Build history of the part. All positions in model axes, mm. Round coordinates to 2 decimals unless told otherwise and drop trailing zeros. Order: outer loops, then holes, each group sorted by start corner. A loop starts at its lowest first (then second) coordinate and runs counter-clockwise, first axis right, second up. Notation, with made-up numbers: M -27.75,42.25 L -6.75,42.25 A23 cw -6.75,67.25 Z; hole C 18.5,-8 d8. An arc over 180 degrees is marked long. One line per item, written item: value. Start each with the question number.
Item 1: Band-saw the part on B-B, the plane y = -2.25. Write the cut outline in (x, z), then the cut area to 3 significant figures.
Item 2: Probe L1, parallel to X at y = 2.5, z = 2.75; L2, parallel to X at y = 2.5, z = 0; L3, parallel to Y at x = -7.75, z = -4. List the from-to ranges inside material, lowest first.
Item 3: Pin check, flat tips, straight feed: pin 1 (1.5 mm diameter, centred on x = 5, y = 2, fed in from -Z); pin 2 (1.5 mm diameter, centred on y = 0, z = 6.5, fed in from +X); pin 3 (4 mm diameter, centred on x = 3.5, y = 2.5, fed in from +Z). Stop position of each tip, or through.
Item 4: Band-saw the part on A-A, the plane y = -0.5. Write the cut outline in (x, z), then the cut area to 3 significant figures.
Item 5: Two-plate mould, pull along Z, no slides. Class faces 1 (the flat face through (-4.6, 3.5, 7.5)), 2 (the cylindrical face through (-2.58, 2.51, -8.18)): +Z half, -Z half, draft (parallel to the pull), parting line (faces both ways), or undercut.
```python
from build123d import *

# Parameters (mm, degrees)
CUT_EXTRUDE1_DEPTH      = 16.720209922
CUT_EXTRUDE1_DEPTH_BACK = 16.720209922
SKETCH3_W               = 21.5
SKETCH3_H               = 0.5


with BuildPart() as part:
    # Sketch2 → Revolve1 (revolve)
    with BuildSketch(Plane.XY, mode=Mode.PRIVATE) as revolve1_sk:
        with BuildLine():
            Line((8.578101022, -1.538329541), (8.578101022, -4))
            Line((8.578101022, -4), (9.978101022, -4))
            ThreePointArc((9.978101022, -4), (10.75, 0), (9.978101022, 4))
            Line((9.978101022, 4), (8.578101022, 4))
            Line((8.578101022, 4), (8.578101022, 1.538329541))
            ThreePointArc((8.578101022, 1.538329541), (9.110552684, 0.849646384), (9.3, 0))
            ThreePointArc((9.3, 0), (9.110552684, -0.849646384), (8.578101022, -1.538329541))
        make_face()
    revolve(revolve1_sk.sketch.rotate(Axis((0, 0, 0), (0, 1, 0)), 90), axis=Axis((0, 0, 0), (0, 1, 0)))

    # Sketch3 → Cut-Extrude1 (cut, two sides: drawn at the far end of the back side and taken through both)
    with BuildSketch(Plane.XY.offset(-CUT_EXTRUDE1_DEPTH_BACK)):
        with Locations((0, 3.75)):
            Rectangle(SKETCH3_W, SKETCH3_H)
        with Locations((0, -3.75)):
            Rectangle(SKETCH3_W, SKETCH3_H)
    extrude(amount=CUT_EXTRUDE1_DEPTH + CUT_EXTRUDE1_DEPTH_BACK, mode=Mode.SUBTRACT)


solid = part.part
```
Output:
1. outline: C 0,0 d21.02; hole C 0,0 d17.16
1. area: 116 mm²
2. L1: x = -10.09 to -8.13, 8.13 to 10.09
2. L2: x = -10.46 to -8.58, 8.58 to 10.46
2. L3: y = -3.5 to -1.41, 1.41 to 3.5
3. pin 1: stops at z = -9.7
3. pin 2: stops at x = 9.08
3. pin 3: stops at z = 10.5
4. outline: C 0,0 d21.48; hole C 0,0 d18.47
4. area: 94.2 mm²
5. face 1: draft
5. face 2: undercut
